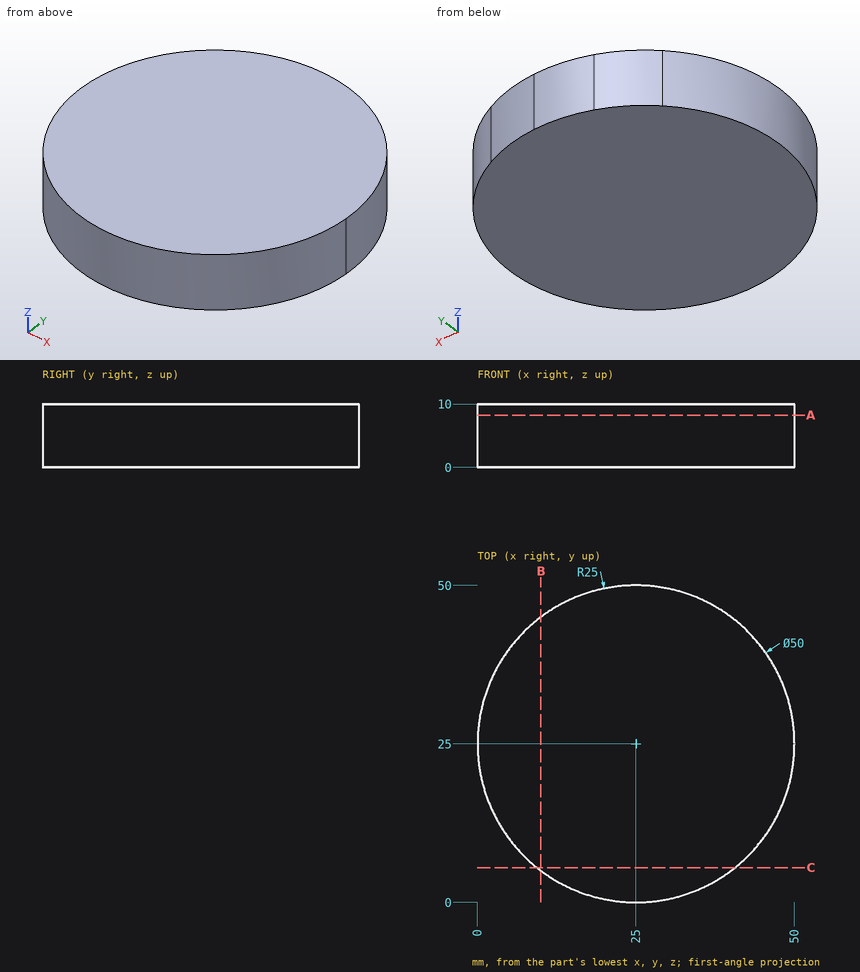
Job drawing, mm, ordinate dimensions from the low corner. One solid piece. Coordinates: 2 decimals unless noted, no trailing zeros. Order: outer loops, then holes, each group sorted by start corner. A loop starts at its lowest first (then second) coordinate and runs counter-clockwise, first axis right, second up. Notation, with made-up numbers: (31.5, 87.5) - (63.5, 87.5) arc R21 ccw to (63.5, 98.5) - close; hole circle Ø3 at (78.5, 58). An arc over 180 degrees is marked (long way). Return JSON: item names as keys, results as strings. Group by question number.
1) Saw through at A-A, the plane z = 8.25. Write the cut outline in (x, y).
2) Probe line 1 (Y direction, x = 24.5, z = 2.5) (3 decimals); line 2 (X direction, y = 48, z = 3.25); line 3 (X direction, y = 25, z = 8.75). List the from-to ranges inside material, lowest first. Write a range as from..to.
3) Saw through at B-B, the plane x = 10. Write the cut outline in (y, z).
4) Saw through at C-C, the plane y = 5.5. Write the cut outline in (x, z), plus the area to 3 significant figures.
5) Flat gauge pins, fed straight in: P1, Ø1, axis at x = 26, z = 4, coming from the -Y side (3 decimals); P2, Ø5, axis at y = 38, z = 8, coming from the -X side; P3, Ø6, axis at x = 35.5, z = 4, coming from the +Y side. Where does each tip first touch, or does it go through?
Values found:
{
 "1": {"outline": "(6.97, 42.32) arc R25 ccw (long way) to (34.8, 48) arc R25 ccw to (25, 50) arc R25 ccw to (15.2, 48) arc R25 ccw to start"},
 "2": {"line 1": "y = 0.005..49.995", "line 2": "x = 15.2..34.8", "line 3": "x = 0..50"},
 "3": {"outline": "(5, 0) - (45, 0) - (45, 10) - (5, 10) - close"},
 "4": {"outline": "(9.36, 0) - (40.64, 0) - (40.64, 10) - (9.36, 10) - close", "area": "313 mm²"},
 "5": {"P1": "stops at y = 0.005", "P2": "stops at x = 2.31", "P3": "stops at y = 48.85"}
}
